CAD build for the part. Positions are in the model's coordinates, mm. A direction names the side the tool comes from. Round coordinates to 2 decimals unless told otherwise and drop trailing zeros. Order: outer loops, then holes, each group sorted by start corner. A loop starts at its lowest first (then second) coordinate and runs counter-clockwise, first axis right, second up.
```python
from build123d import *

# Parameters (mm, degrees)
F1_DEPTH  = 7.5
F2_R      = 32.7718142907
F3_DEPTH  = 8
F4_W      = 0.75
F4_H      = 80
F5_DEPTH  = 7.5
F6_R      = 2.7597283283
F7_DEPTH  = 25
F8_R      = 2.75
F9_DEPTH  = 25
F11_START = -10
F10_R     = 4.7926746231
F11_DEPTH = 12


with BuildPart() as f1:
    # F0 (on Top) → F1 (new body, symmetric)
    with BuildSketch(Plane.XY):
        with BuildLine():
            Line((0, 42.5), (-32.5, 42.5))
            ThreePointArc((-32.5, 42.5), (-39.5710678119, 39.5710678119), (-42.5, 32.5))
            Line((-42.5, 32.5), (-42.5, 0))
            Line((-42.5, 0), (-42.5, -22.5))
            ThreePointArc((-42.5, -22.5), (-36.6421356237, -36.6421356237), (-22.5, -42.5))
            Line((-22.5, -42.5), (-14.2230435639, -42.5))
            ThreePointArc((-14.2230435639, -42.5), (-12.1017232203, -43.3786796564), (-11.2230435639, -45.5))
            Line((-11.2230435639, -45.5), (-11.2230435639, -55.5))
            ThreePointArc((-11.2230435639, -55.5), (-10.3443639075, -57.6213203436), (-8.2230435639, -58.5))
            Line((-8.2230435639, -58.5), (9.5, -58.5))
            ThreePointArc((9.5, -58.5), (11.6213203436, -57.6213203436), (12.5, -55.5))
            Line((12.5, -55.5), (12.5, -45.5))
            ThreePointArc((12.5, -45.5), (13.3786796564, -43.3786796564), (15.5, -42.5))
            Line((15.5, -42.5), (22.5, -42.5))
            ThreePointArc((22.5, -42.5), (36.6421356237, -36.6421356237), (42.5, -22.5))
            Line((42.5, -22.5), (42.5, 0))
            Line((42.5, 0), (42.5, 32.5))
            ThreePointArc((42.5, 32.5), (39.5710678119, 39.5710678119), (32.5, 42.5))
            Line((32.5, 42.5), (0, 42.5))
        make_face()
    extrude(amount=F1_DEPTH, both=True)

    # F2 (on Top) → F3 (cut, symmetric)
    with BuildSketch(Plane.XY):
        Circle(F2_R)
    extrude(amount=F3_DEPTH, both=True, mode=Mode.SUBTRACT)

    # F4 (on Top) → F5 (cut, symmetric)
    with BuildSketch(Plane.XY):
        with Locations((0.375, -40)):
            Rectangle(F4_W, F4_H)
        with Locations((-0.375, -40)):
            Rectangle(F4_W, F4_H)
    extrude(amount=F5_DEPTH, both=True, mode=Mode.SUBTRACT)

    # F6 (on Right) → F7 (cut, symmetric)
    with BuildSketch(Plane.YZ):
        with Locations((-50.511858446, 0)):
            Circle(F6_R)
    extrude(amount=F7_DEPTH, both=True, mode=Mode.SUBTRACT)

    # F8 (on face) → F9 (cut)
    with BuildSketch(Plane(origin=(0, 42.5, 0), x_dir=(-1, 0, 0), z_dir=(0, 1, 0))):
        with Locations((20, 0)):
            Circle(F8_R)
        with Locations((-20, 0)):
            Circle(F8_R)
    extrude(amount=-F9_DEPTH, mode=Mode.SUBTRACT)

    # F10 (on face) → F11 (cut)
    with BuildSketch(Plane(origin=(0, 42.5, 0), x_dir=(-1, 0, 0), z_dir=(0, 1, 0)).offset(F11_START)):
        with Locations((20, 0)):
            Circle(F10_R)
        with Locations((-20, 0)):
            Circle(F10_R)
    extrude(amount=-F11_DEPTH, mode=Mode.SUBTRACT)


solid = f1.part
```
1. Cut at A-A, the plane x = -3. Write the cut outline in (y, z).
2. Cut at B-B, the plane y = -34. Write the cut outline in (x, z), and give its area (3 significant figures).
3. Mould opens along Z. For faces 4 (the face through (6.71, -53.27, 0.12)), 5 (the face through (42.5, 5, 0)) say: released by +Z, released by -Z, zero draft, split by the parting line, or undercut.
4. Cut at C-C, the plane x = 20. Write the cut outline in (y, z).
5. Cut at D-D, the plane z = 6. Write the cut outline in (x, y), and give its area (3 significant figures).
6. Pin check, flat tips, straight feed: P1, Ø3, axis at x = 18, z = -2, coming from the -Y side; P2, Ø4.5, axis at y = -40.5, z = 3, coming from the -X side; P3, Ø6.5, axis at x = -16.5, z = 2, coming from the -Y side. Stop position of each tip, or through.
7. Drill centre lines: line 1 (X direction, y = 23.75, z = 0); line 2 (Y direction, x = 4, z = -5); line 3 (Z direction, x = 20, y = 27.5). Where is each one in solid material? Low to high.
8. Tool access for faces 1 (the face through (12.5, -53, 2)), 2 (the face through (-0.75, -46, 0)), 3 (the face through (22.747, 37.57, 0.121)): list every direction of +Z, -Z, +X, -X, +Y, -Y with a clear straight run to the whole face (end or side of a thin tool).
Outcome:
1. outline: (-58.5, -7.5) - (-32.63, -7.5) - (-32.63, 7.5) - (-58.5, 7.5) - close; (32.63, -7.5) - (42.5, -7.5) - (42.5, 7.5) - (32.63, 7.5) - close; hole circle Ø5.52 at (-50.51, 0)
2. outline: (-38.86, -7.5) - (-0.75, -7.5) - (-0.75, 7.5) - (-38.86, 7.5) - close; (0.75, -7.5) - (38.86, -7.5) - (38.86, 7.5) - (0.75, 7.5) - close
2. area: 1,140 mm2
3. face 4: undercut
3. face 5: zero draft
4. outline: (-42.5, -7.5) - (-25.96, -7.5) - (-25.96, 7.5) - (-42.5, 7.5) - close; (25.96, -7.5) - (42.5, -7.5) - (42.5, -2.75) - (32.5, -2.75) - (32.5, -4.79) - (25.96, -4.79) - close; (25.96, 4.79) - (32.5, 4.79) - (32.5, 2.75) - (42.5, 2.75) - (42.5, 7.5) - (25.96, 7.5) - close
5. outline: (-42.5, -22.5) arc R20 ccw to (-22.5, -42.5) - (-14.22, -42.5) arc R3 cw to (-11.22, -45.5) - (-11.22, -55.5) arc R3 ccw to (-8.22, -58.5) - (-0.75, -58.5) - (-0.75, -32.76) arc R32.77 cw (long way) to (0.75, -32.76) - (0.75, -58.5) - (9.5, -58.5) arc R3 ccw to (12.5, -55.5) - (12.5, -45.5) arc R3 cw to (15.5, -42.5) - (22.5, -42.5) arc R20 ccw to (42.5, -22.5) - (42.5, 32.5) arc R10 ccw to (32.5, 42.5) - (-32.5, 42.5) arc R10 ccw to (-42.5, 32.5) - close
5. area: 3,980 mm2
6. P1: stops at y = -42.5
6. P2: stops at x = -34.83
6. P3: stops at y = -42.66
7. line 1: x = -42.5 to -24.79, 24.79 to 42.5
7. line 2: y = -58.5 to -32.53, 32.53 to 42.5
7. line 3: z = -7.5 to -4.79, 4.79 to 7.5
8. face 1: +Z, -Z, +X, -Y
8. face 2: +Z, -Z, -Y
8. face 3: +Y
